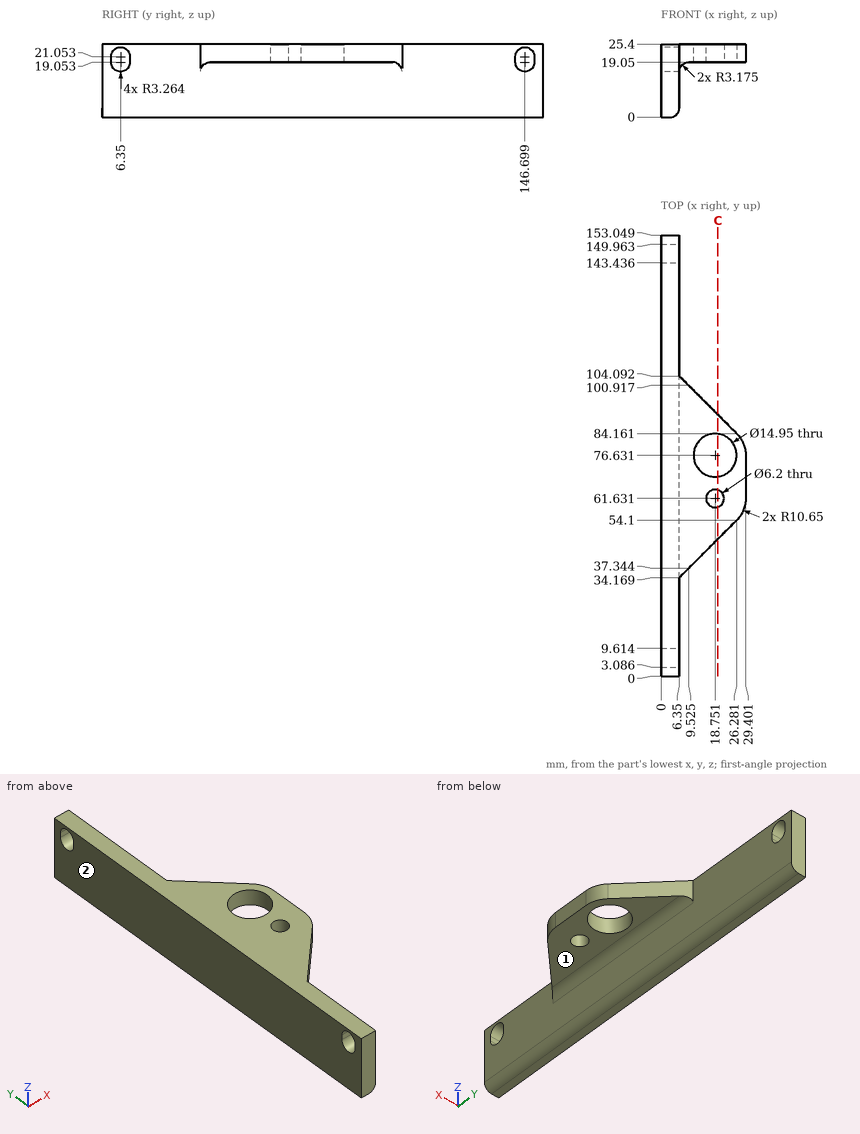
The drawing under review shows one solid part. Ordinate dimensions are in mm from its lowest x, y, z. A direction names the side the tool comes from. Give positions to 0.01 mm unless a question says otherwise; leave off trailing zeros. Write item = value, one per line. Start each with the question number.
(1) For the marked faces 1 and 2, list the 3-axis set-ups (+Z, -Z, +X, -X, +Y, -Y) from which the entire face can be reached by the end or side of a thin tool; tool diameter is ignored.
(2) For pin 1 (4 mm diameter, centred on y = 93, z = 6, fed in from +X); pin 2 (2 mm diameter, centred on y = 106.5, z = 16.5, fed in from +X); pin 3 (10 mm diameter, centred on x = 18.5, y = 55.5, fed in from -Z), all flat-tipped, find the tip position at first contact; note any pin that passes through.
(3) We need section C-C on x = 19.75. State how many separate pieces and enclosed holes the cut face has.
(4) To check wall thickness, follow line 1 along X through (y, z) = (106, 5.25); line 2 along Z through (x, y) = (9.5, 71). State the ranges of each line that lie inside material, in increasing order.
Numbers:
q1.face_1 = -Z, +X, +Y, -Y
q1.face_2 = +Z, -Z, -X, +Y, -Y
q2.pin_1 = 6.35
q2.pin_2 = 6.35
q2.pin_3 = 19.05
q3.separate_pieces = 3
q3.enclosed_holes = 0
q4.line_1 = 0 to 6.35
q4.line_2 = 19.05 to 25.4
